from build123d import *

# Parameters (mm, degrees)
BOSS_EXTRUDE2_DEPTH = 29.21
SKETCH2_W           = 22.352
SKETCH2_H           = 25.4
BOSS_EXTRUDE3_DEPTH = 3.81
SKETCH5_R           = 11.176
BOSS_EXTRUDE6_DEPTH = 25.4


with BuildPart() as part:
    # Sketch1 → Boss-Extrude2 (new body)
    with BuildSketch(Plane.XY):
        Polygon((-12.043317073, 53.947940362), (15.134682927, 53.947940362), (15.134682927, -17.934059638), (-51.921317073, -17.934059638), (-51.921317073, 53.947940362), (-24.743317073, 53.947940362), (-24.743317073, 37.945940362), (-50.143317073, 37.945940362), (-50.143317073, -0.154059638), (13.356682927, -0.154059638), (13.356682927, 37.945940362), (-12.043317073, 37.945940362), align=None)
    extrude(amount=BOSS_EXTRUDE2_DEPTH)

    # Sketch2 → Boss-Extrude3 (add)
    with BuildSketch(Plane.XY.offset(29.21)):
        with Locations((-18.393317073, -30.634059638)):
            Rectangle(SKETCH2_W, SKETCH2_H)
    extrude(amount=-BOSS_EXTRUDE3_DEPTH)

    # Sketch5 → Boss-Extrude6 (add)
    with BuildSketch(Plane.XY.offset(29.21)):
        with Locations((-18.393317073, -43.334059638)):
            Circle(SKETCH5_R)
    extrude(amount=-BOSS_EXTRUDE6_DEPTH)


solid = part.part
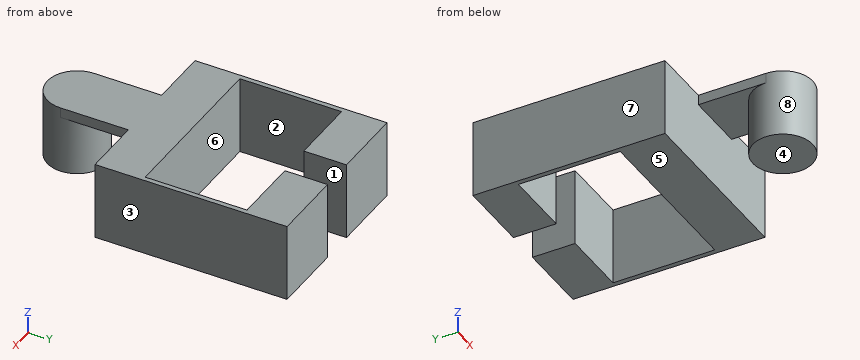
CAD build for the part. Positions are in the model's coordinates, mm. Face numbers are marked on the shaded views. A direction names the side the tool comes from. Give positions to 0.01 mm unless a question says otherwise; leave off trailing zeros. Write each loop counter-clockwise with the first axis right and the second up, starting at its lowest first coordinate (ties: lowest second). Pieces come first, ordered by that corner, then holes. Notation, with made-up numbers: (0.5, 79.25) -> (35.5, 79.25) arc R30 cw to (35.5, 106.25) -> close; hole circle Ø3 at (34.5, -14.5). An arc over 180 degrees is marked (long way). Return JSON: item names as keys, results as strings.
Item 1: Band-saw the part on B-B (y = 30). List the corners of the cut face in (x, z), then the cut area to 3 significant figures.
Answer below:
{"outline": "(-51.92, 0) -> (-50.14, 0) -> (-50.14, 29.21) -> (-51.92, 29.21) -> close; (13.36, 0) -> (15.13, 0) -> (15.13, 29.21) -> (13.36, 29.21) -> close", "area": "104 mm2"}
Item 2: Two-plate mould, pull along X, no slides. Class the marked faces 5, 6, 7 and 8: +X half, -X half, draft (parallel to the pull), parting line (faces both ways), or undercut.
Answer below:
{"face 5": "draft", "face 6": "undercut", "face 7": "-X half", "face 8": "parting line"}
Item 3: Band-saw the part on C-C (z = 17.75). List the corners of the cut face in (x, y), then the cut area to 3 significant figures.
Answer below:
{"outline": "(-51.92, -17.93) -> (15.13, -17.93) -> (15.13, 53.95) -> (-12.04, 53.95) -> (-12.04, 37.95) -> (13.36, 37.95) -> (13.36, -0.15) -> (-50.14, -0.15) -> (-50.14, 37.95) -> (-24.74, 37.95) -> (-24.74, 53.95) -> (-51.92, 53.95) -> close; circle Ø22.35 at (-18.39, -43.33)", "area": "2,590 mm2"}
Item 4: Band-saw the part on D-D (y = -29). List the corners of the cut face in (x, z), then the cut area to 3 significant figures.
Answer below:
{"outline": "(-29.57, 25.4) -> (-7.22, 25.4) -> (-7.22, 29.21) -> (-29.57, 29.21) -> close", "area": "85.2 mm2"}
Item 5: Drop flat-ended pins along their axis: pin 1 (3 mm diameter, centred on x = -13.5, z = 21.5, fed in from -Y); pin 2 (12.5 mm diameter, centred on x = -0.5, z = 11, fed in from -Y); pin 3 (4 mm diameter, centred on y = -24.5, z = 28, fed in from -X). Give the stop position or say it passes through.
Answer below:
{"pin 1": "stops at y = -53.98", "pin 2": "stops at y = -17.93", "pin 3": "stops at x = -29.57"}
Item 6: Band-saw the part on A-A (x = -6). List the corners of the cut face in (y, z), then the cut area to 3 significant figures.
Answer below:
{"outline": "(-17.93, 0) -> (-0.15, 0) -> (-0.15, 29.21) -> (-17.93, 29.21) -> close; (37.95, 0) -> (53.95, 0) -> (53.95, 29.21) -> (37.95, 29.21) -> close", "area": "987 mm2"}
Item 7: Tool access for the marked faces 1, 2, 3 and 4: list every direction of +Z, -Z, +X, -X, +Y, -Y with a clear straight run to the whole face (end or side of a thin tool).
Answer below:
{"face 1": "+Z, -Z, +Y", "face 2": "+Z, -Z", "face 3": "+Z, -Z, +X, +Y, -Y", "face 4": "-Z, +X, -X, -Y"}
Item 8: Drill centre lines: probe 1 along X at (y, z) = (10, 24.25); probe 2 along Y at (x, z) = (11, 5.25); probe 3 along X at (y, z) = (39, 11.5). Where is each one in solid material? Low to high.
Answer below:
{"probe 1": "x = -51.92 to -50.14, 13.36 to 15.13", "probe 2": "y = -17.93 to -0.15, 37.95 to 53.95", "probe 3": "x = -51.92 to -24.74, -12.04 to 15.13"}
